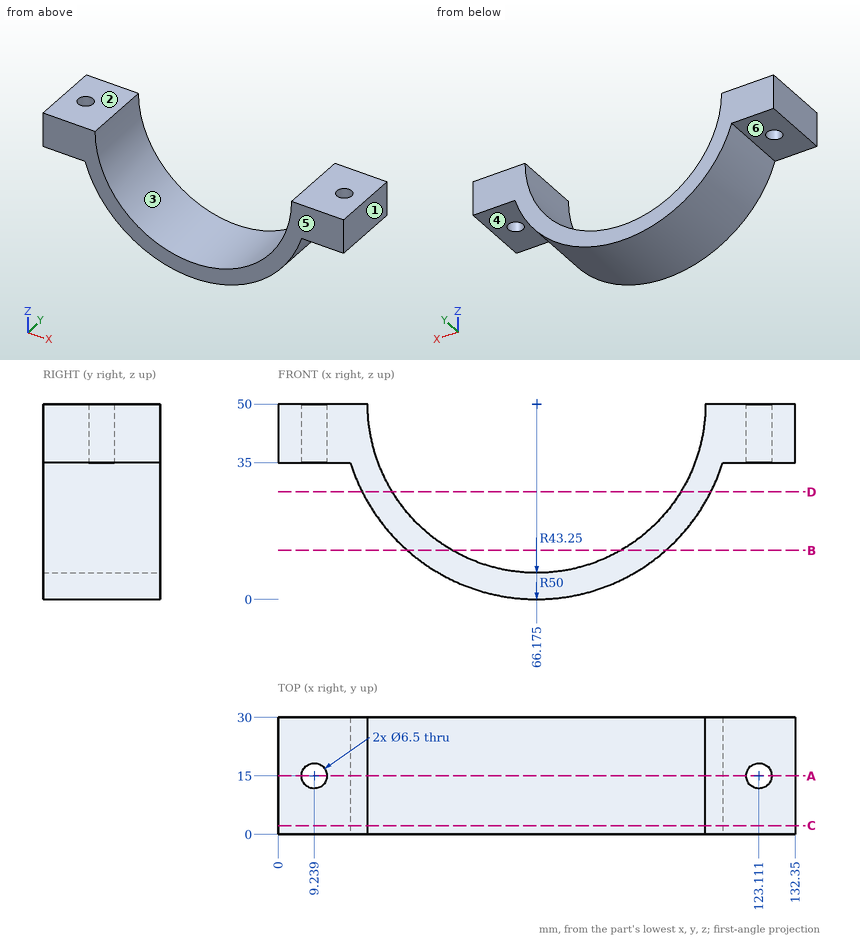
For this review, use the dimensioned drawing (mm, ordinates from the lowest corner) and the shaded views. A direction names the side the tool comes from. Round coordinates to 2 decimals unless told otherwise and drop trailing zeros. Order: outer loops, then holes, each group sorted by start corner. A loop starts at its lowest first (then second) coordinate and runs counter-clockwise, first axis right, second up. Notation, with made-up numbers: (77, -11.5) -> (134, -11.5) arc R22 ccw to (134, 12.5) -> close; hole circle Ø11 at (21.5, 61). An arc over 180 degrees is marked (long way). Use CSV: the item, a comma, the result in double quotes. Start each with the question number.
(1) Wall thickness on probe 1 along X at (y, z) = (27.5, 46); probe 2 along X at (y, z) = (16.75, 40); probe 3 along X at (y, z) = (18, 17.5): over which ranges is each line inside the solid? List them lowest first. Write a range as from..to.
(2) Mouldability with a two-part tool opening along X and no side actions: class the marked faces 1, 2 and 3 as pulls with the +X half, pulls with the -X half, needs draft (parallel to the pull), parting line crosses it, or undercut.
(3) Consider section A-A on y = 15. Write out the cut boundary in (x, z) (3 decimals), and give its area (3 significant figures).
(4) Consider section D-D on z = 27.5. Write out the cut boundary in (x, y), and give its area (3 significant figures).
(5) Consider section C-C on y = 2.25. Write out the cut boundary in (x, z) (3 decimals), and give its area (3 significant figures).
(6) Insertion check: pin 1 (1.5 mm diameter, centred on y = 4.5, z = 6, fed in from +X); pin 2 (8 mm diameter, centred on x = 70, y = 19, fed in from +Z); pin 3 (8.5 mm diameter, centred on x = 9.24, y = 15, fed in from +Z); pin 4 (9 mm diameter, centred on x = 124.5, y = 14, fed in from -Z). Each pin has a flat end and moves straight along its axis. Give the tip position at first contact, or say it passes through.
(7) Tool access review of the marked faces 4, 5 and 6: name each direction out of +Z, -Z, +X, -X, +Y, -Y from which nothing blocks a thin tool from reaching the whole face with its end or side.
(8) Consider section B-B on z = 12.5. Write out the cut boundary in (x, y).
Responses:
1,probe 1,"0..23.11, 109.24..132.35"
1,probe 2,"0..6.5, 11.98..24.1, 108.25..120.37, 125.85..132.35"
1,probe 3,"28.18..37.64, 94.71..104.17"
2,face 1,"pulls with the +X half"
2,face 2,"needs draft"
2,face 3,"undercut"
3,outline,"(0, 35) -> (5.989, 35) -> (5.989, 50) -> (0, 50) -> close; (12.489, 35) -> (18.478, 35) arc R50 ccw to (113.872, 35) -> (119.861, 35) -> (119.861, 50) -> (109.425, 50) arc R43.25 cw to (22.925, 50) -> (12.489, 50) -> close; (126.361, 35) -> (132.35, 35) -> (132.35, 50) -> (126.361, 50) -> close"
3,area,"1,300 mm²"
4,outline,"(21.52, 0) -> (29.24, 0) -> (29.24, 30) -> (21.52, 30) -> close; (103.11, 0) -> (110.83, 0) -> (110.83, 30) -> (103.11, 30) -> close"
4,area,"463 mm²"
5,outline,"(0, 35) -> (18.478, 35) arc R50 ccw to (113.872, 35) -> (132.35, 35) -> (132.35, 50) -> (109.425, 50) arc R43.25 cw to (22.925, 50) -> (0, 50) -> close"
5,area,"1,500 mm²"
6,pin 1,"x = 91.26"
6,pin 2,"z = 7.46"
6,pin 3,"z = 50"
6,pin 4,"z = 35"
7,face 4,"-Z, +X, +Y, -Y"
7,face 5,"+Z, -Z, +X, -X, -Y"
7,face 6,"-Z, -X, +Y, -Y"
8,outline,"(33.1, 0) -> (44.63, 0) -> (44.63, 30) -> (33.1, 30) -> close; (87.72, 0) -> (99.25, 0) -> (99.25, 30) -> (87.72, 30) -> close"
